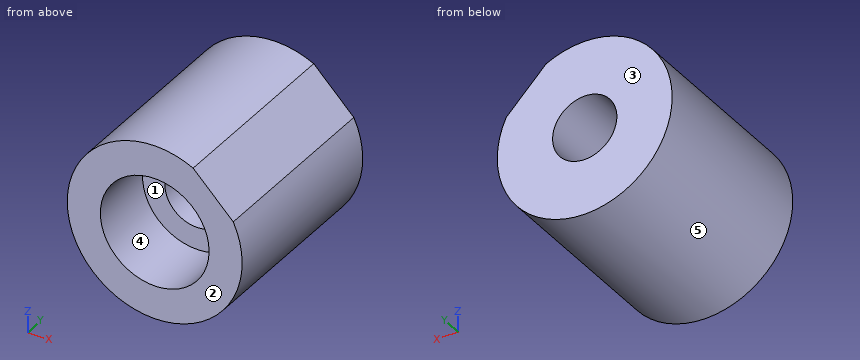
```python
from build123d import *

# Parameters (mm, degrees)
F0_R     = 4.699
F0_R_2   = 1.7272
F1_DEPTH = 10.16
F3_DEPTH = 10.161
F4_R     = 2.921
F4_R_2   = 1.7272
F4_R_3   = 1.7145
F5_DEPTH = 3.556


with BuildPart() as f1:
    # F0 (on Front) → F1 (new body)
    with BuildSketch(Plane.XZ):
        Circle(F0_R)
        Circle(F0_R_2, mode=Mode.SUBTRACT)
    extrude(amount=F1_DEPTH)

    # F2 (on face) → F3 (cut, through all)
    with BuildSketch(Plane.XZ.offset(10.16)):
        with BuildLine():
            ThreePointArc((4.2207203769, 2.0654589078), (3.3226947648, 3.3226947648), (2.0654589078, 4.2207203769))
            Line((2.0654589078, 4.2207203769), (4.2207203769, 2.0654589078))
        make_face()
    extrude(amount=-F3_DEPTH, mode=Mode.SUBTRACT)

    # F4 (on face) → F5 (cut)
    with BuildSketch(Plane.XZ.offset(10.16)):
        Circle(F4_R)
        Circle(F4_R_2, mode=Mode.SUBTRACT)
        Circle(F4_R_2)
        Circle(F4_R_3, mode=Mode.SUBTRACT)
    extrude(amount=-F5_DEPTH, mode=Mode.SUBTRACT)


solid = f1.part
```
Could you check a few things on this model? Use its own coordinates, in mm. Face numbers are marked on the shaded views. A direction names the side the tool comes from. Coordinates: 2 decimals unless noted, no trailing zeros. Write each loop counter-clockwise with the first axis right and the second up, starting at its lowest first coordinate (ties: lowest second). Pieces come first, ordered by that corner, then holes. Notation, with made-up numbers: (78, 20) -> (117, 20) arc R21 ccw to (117, 46) -> close; hole circle Ø2 at (20, -3.75). An arc over 180 degrees is marked (long way). Return JSON: item names as keys, results as strings.
(1) We'd pull the mould along Z, two halves only. Please class the marked faces 3, 4 and 5: +Z half, -Z half, draft (parallel to the pull), parting line (faces both ways), or undercut.
Numbers:
{"face 3": "draft", "face 4": "undercut", "face 5": "parting line"}
(2) Imagine slicing it at B-B, the plane z = 0. Please give me the cut outline in (x, y), then the cut area to 3 significant figures.
Numbers:
{"outline": "(-4.7, -10.16) -> (-2.92, -10.16) -> (-2.92, -6.6) -> (-1.73, -6.6) -> (-1.73, 0) -> (-4.7, 0) -> close; (1.73, -6.6) -> (2.92, -6.6) -> (2.92, -10.16) -> (4.7, -10.16) -> (4.7, 0) -> (1.73, 0) -> close", "area": "51.9 mm2"}
(3) I'm going to push flat-ended pins straight in: pin 1 (4 mm diameter, centred on x = 3.5, y = -1.5, fed in from +Z); pin 2 (2 mm diameter, centred on x = -0.5, z = 1.5, fed in from -Y); pin 3 (5 mm diameter, centred on x = 3.5, y = -7.5, fed in from +Z). Where does each tip first touch, or does it pass through?
Numbers:
{"pin 1": "stops at z = 4.45", "pin 2": "stops at y = -6.6", "pin 3": "stops at z = 4.59"}
(4) Imagine slicing it at A-A, the plane x = 0. Please give me the cut outline in (y, z).
Numbers:
{"outline": "(-10.16, -4.7) -> (0, -4.7) -> (0, -1.73) -> (-6.6, -1.73) -> (-6.6, -2.92) -> (-10.16, -2.92) -> close; (-10.16, 2.92) -> (-6.6, 2.92) -> (-6.6, 1.73) -> (0, 1.73) -> (0, 4.7) -> (-10.16, 4.7) -> close"}
(5) Imagine slicing it at C-C, the plane y = -3. Please give me the cut outline in (x, z), then the cut area to 3 significant figures.
Numbers:
{"outline": "(2.07, 4.22) arc R4.7 ccw (long way) to (4.22, 2.07) -> close; hole circle Ø3.45 at (0, 0)", "area": "59.5 mm2"}
(6) Which directions (+Z, -Z, +X, -X, +Y, -Y) give clear straight access to the entire face, cutting with the end or side of a thin tool? Please do the marked faces 1 and 2.
Numbers:
{"face 1": "-Y", "face 2": "+Z, -Z, +X, -X, -Y"}
(7) I need wall thicknesses on L1, parallel to Z at x = 0, y = -1.5; L2, parallel to Z at x = 0, y = -8.4. Which ranges of each line are inside material? Lowest first, please.
Numbers:
{"L1": "z = -4.7 to -1.73, 1.73 to 4.7", "L2": "z = -4.7 to -2.92, 2.92 to 4.7"}
(8) Imagine slicing it at D-D, the plane z = -2. Please give me the cut outline in (x, y).
Numbers:
{"outline": "(-4.25, -10.16) -> (-2.13, -10.16) -> (-2.13, -6.6) -> (2.13, -6.6) -> (2.13, -10.16) -> (4.25, -10.16) -> (4.25, 0) -> (-4.25, 0) -> close"}
